Build history of the part. All positions in model axes, mm. Coordinates: 2 decimals unless noted, no trailing zeros. Write item = value, one per line. Start each with the question number.
Q1. Drill centre lines: probe 1 along Z at (x, y) = (63.5, 3.25); probe 2 along Z at (x, y) = (100.5, 1). Where is each one in solid material? Low to high.
Q2. Band-saw the part on A-A on y = 2. State how many separate pieces and enclosed holes the cut face has, plus the area to 3 significant figures.
Q3. Pin check, flat tips, straight feed: P1, Ø5.5, axis at x = 127, z = -12.7, coming from the -Y side; P2, Ø4, axis at x = 254, z = -12.7, coming from the +Y side. Stop position of each tip, or through.
```python
from build123d import *

# Parameters (mm, degrees)
SKETCH1_W               = 406.4
SKETCH1_H               = 25.4
BOSS_EXTRUDE1_DEPTH     = 6.35
SKETCH2_R               = 2.4892
CUT_EXTRUDE1_DEPTH      = 1
CUT_EXTRUDE1_DEPTH_BACK = 7.35
SKETCH3_R               = 2.378070279
SKETCH3_R_2             = 2.20737703
CUT_EXTRUDE2_DEPTH      = 7.35


with BuildPart() as part:
    # Sketch1 → Boss-Extrude1 (new body)
    with BuildSketch(Plane(origin=(0, 0, 0), x_dir=(1, 0, 0), z_dir=(0, 1, 0))):
        with Locations((203.2, 12.7)):
            Rectangle(SKETCH1_W, SKETCH1_H)
    extrude(amount=BOSS_EXTRUDE1_DEPTH)

    # Sketch2 → Cut-Extrude1 (cut, two sides)
    with BuildSketch(Plane(origin=(0, 6.35, 0), x_dir=(1, 0, 0), z_dir=(0, 1, 0))) as cut_extrude1_sk:
        with Locations((381, 12.7)):
            Circle(SKETCH2_R)
        with Locations((355.6, 12.7)):
            Circle(SKETCH2_R)
        with Locations((330.2, 12.7)):
            Circle(SKETCH2_R)
        with Locations((304.8, 12.7)):
            Circle(SKETCH2_R)
        with Locations((279.4, 12.7)):
            Circle(SKETCH2_R)
        with Locations((254, 12.7)):
            Circle(SKETCH2_R)
        with Locations((228.6, 12.7)):
            Circle(SKETCH2_R)
        with Locations((203.2, 12.7)):
            Circle(SKETCH2_R)
        with Locations((177.8, 12.7)):
            Circle(SKETCH2_R)
        with Locations((152.4, 12.7)):
            Circle(SKETCH2_R)
        with Locations((127, 12.7)):
            Circle(SKETCH2_R)
        with Locations((101.6, 12.7)):
            Circle(SKETCH2_R)
    extrude(amount=CUT_EXTRUDE1_DEPTH, mode=Mode.SUBTRACT)
    extrude(cut_extrude1_sk.sketch, amount=-CUT_EXTRUDE1_DEPTH_BACK, mode=Mode.SUBTRACT)

    # Sketch3 → Cut-Extrude2 (cut, through all)
    with BuildSketch(Plane.XZ):
        with Locations((63.5, -12.7)):
            Circle(SKETCH3_R)
        with Locations((38.1, -12.7)):
            Circle(SKETCH3_R_2)
    extrude(amount=-CUT_EXTRUDE2_DEPTH, mode=Mode.SUBTRACT)


solid = part.part
```
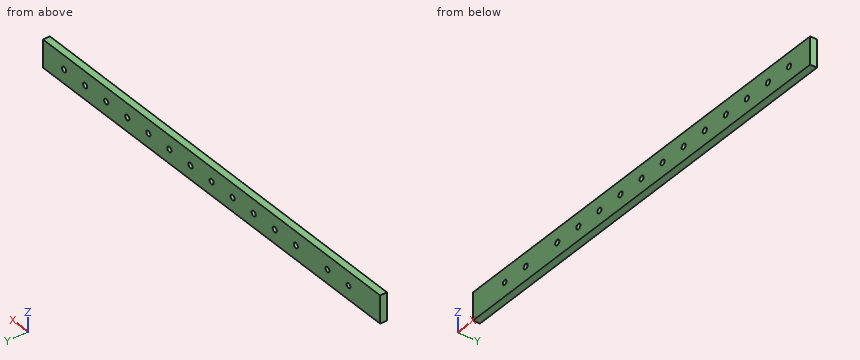
Recorded:
q1.probe_1 = -25.4 to -15.08, -10.32 to 0
q1.probe_2 = -25.4 to -14.93, -10.47 to 0
q2.separate_pieces = 1
q2.enclosed_holes = 14
q2.area = 10,100 mm2
q3.P1 = 0
q3.P2 = through
